Read the model definition and answer for the solid it produces. Units are mm, in the model's axes. A direction names the side the tool comes from. Round coordinates to 2 decimals unless told otherwise and drop trailing zeros. Write each loop counter-clockwise with the first axis right and the second up, starting at its lowest first coordinate (ties: lowest second). Pieces come first, ordered by that corner, then holes. Notation, with made-up numbers: (27, -11) -> (82, -11) arc R34 ccw to (82, 20) -> close; hole circle Ø3 at (54.5, 31.25). An arc over 180 degrees is marked (long way). Return JSON: item names as keys, results as strings.
from build123d import *

# Parameters (mm, degrees)
F0_W     = 139.7
F0_H     = 63.5
F0_W_2   = 115.509763
F0_H_2   = 43.004075
F1_DEPTH = 6.35
F2_W     = 12.7
F2_H     = 63.5
F3_DEPTH = 6.173076
F4_R     = 3.175
F5_DEPTH = 32.64235
F6_W     = 12.237505
F6_H     = 63.5
F7_DEPTH = 6.1722
F8_R     = 3.175
F9_DEPTH = 25.4


with BuildPart() as f1:
    # F0 (on Top) → F1 (new body)
    with BuildSketch(Plane.XY):
        with Locations((-18.169344, -8.735743)):
            Rectangle(F0_W, F0_H)
        with Locations((-17.179944, -7.856222)):
            Rectangle(F0_W_2, F0_H_2, mode=Mode.SUBTRACT)
    extrude(amount=F1_DEPTH)

    # F2 (on face) → F3 (join)
    with BuildSketch(Plane.XZ.offset(40.485743)):
        with Locations((42.790656, 38.1)):
            Rectangle(F2_W, F2_H)
    extrude(amount=-F3_DEPTH)

    # F4 (on face) → F5 (cut)
    with BuildSketch(Plane(origin=(0, -34.312667, 0), x_dir=(-1, 0, 0), z_dir=(0, 1, 0))):
        with Locations((-42.790656, 60.325)):
            Circle(F4_R)
    extrude(amount=-F5_DEPTH, mode=Mode.SUBTRACT)

    # F6 (on face) → F7 (join)
    with BuildSketch(Plane(origin=(0, 23.014257, 0), x_dir=(-1, 0, 0), z_dir=(0, 1, 0))):
        with Locations((-43.021904, 38.1)):
            Rectangle(F6_W, F6_H)
    extrude(amount=-F7_DEPTH)

    # F8 (on face) → F9 (cut)
    with BuildSketch(Plane(origin=(0, 23.014257, 0), x_dir=(-1, 0, 0), z_dir=(0, 1, 0))):
        with Locations((-43.021903, 60.325)):
            Circle(F8_R)
    extrude(amount=-F9_DEPTH, mode=Mode.SUBTRACT)


solid = f1.part
Item 1: Flat-ended cylindrical pins translate along their axes: pin 1 (5 mm diameter, centred on y = 21, z = 45.5, fed in from +X); pin 2 (3 mm diameter, centred on y = 21.5, z = 25, fed in from -X); pin 3 (3 mm diameter, centred on y = -36.5, z = 48, fed in from -X). Find the tip coordinate at first contact, or state that the pin passes through.
Worked answers:
{"pin 1": "stops at x = 49.14", "pin 2": "stops at x = 36.9", "pin 3": "stops at x = 36.44"}
Item 2: Section A-A (y = 3.5) is taken. Give the vertices of the cut face in (x, z), then the cut area to 3 significant figures.
Worked answers:
{"outline": "(-88.02, 0) -> (-74.93, 0) -> (-74.93, 6.35) -> (-88.02, 6.35) -> close; (40.57, 0) -> (51.68, 0) -> (51.68, 6.35) -> (40.57, 6.35) -> close", "area": "154 mm2"}
Item 3: For a pull along Z with two mould halves and no side action, classify faces 5 (the cylindrical face through (41.315, 19.971, 63.002)), 6 (the flat face through (43, -34.313, 39)), 7 (the flat face through (43, 20, 69.85)) as released by +Z, released by -Z, zero draft, split by the parting line, or undercut.
Worked answers:
{"face 5": "undercut", "face 6": "zero draft", "face 7": "released by +Z"}
Item 4: Straight lines are drawn through the part: L1, parallel to Y at x = 37.5, z = 43; L2, parallel to X at y = -17.5, z = 4; L3, parallel to X at y = -37, z = 54. For each, find the intervals that lie inside material, in ascending order. Write a range as [from, to].
Worked answers:
{"L1": "y = [-40.49, -34.31], [16.84, 23.01]", "L2": "x = [-88.02, -74.93], [40.57, 51.68]", "L3": "x = [36.44, 49.14]"}
Item 5: Section B-B (z = 18) is taken. Give the vertices of the cut face in (x, y).
Worked answers:
{"outline": "(36.44, -40.49) -> (49.14, -40.49) -> (49.14, -34.31) -> (36.44, -34.31) -> close; (36.9, 16.84) -> (49.14, 16.84) -> (49.14, 23.01) -> (36.9, 23.01) -> close"}
Item 6: A tool of negligible diameter and unlimited length cuts with its end or side. For faces 1 (the flat face through (36.441, -37, 38)), 2 (the flat face through (36.903, 20, 38)), 3 (the flat face through (49.141, 20, 38)), 4 (the flat face through (-18, 13.646, 3)), from which of +Z, -Z, +X, -X, +Y, -Y can it reach the whole face along a straight path? Write none if from no direction.
Worked answers:
{"face 1": "+Z, -X, +Y, -Y", "face 2": "+Z, -X, +Y", "face 3": "+Z, +X, +Y, -Y", "face 4": "+Z, -Z"}
Item 7: Section C-C (y = 18.5) is taken. Give the vertices of the cut face in (x, z) (3 decimals).
Worked answers:
{"outline": "(-88.019, 0) -> (51.681, 0) -> (51.681, 6.35) -> (49.141, 6.35) -> (49.141, 69.85) -> (36.903, 69.85) -> (36.903, 6.35) -> (-88.019, 6.35) -> close; hole circle Ø6.35 at (43.022, 60.325)"}
